Here's how the part is built. I have some questions about the finished solid (model axes, mm). A direction names the side the tool comes from. Coordinates: 2 decimals unless noted, no trailing zeros. Write each loop counter-clockwise with the first axis right and the second up, starting at its lowest first coordinate (ties: lowest second). Pieces come first, ordered by that corner, then holes. Notation, with made-up numbers: M -17.75,16 L 21.25,16 A33 cw 21.25,48 Z; hole C -17,42 d9. An arc over 180 degrees is marked long. Write each question's results on one line, items separated by ' | '. Start each with the question number.
from build123d import *

# Parameters (mm, degrees)
SKETCH_1_W          = 56.4
SKETCH_1_H          = 56.4
SKETCH_1_R          = 2.5
EXTRUDE_1_DEPTH     = 54.5
SKETCH_2_R          = 4
EXTRUDE_2_DEPTH     = 22
CUT_EXTRUDE_START   = -18
CUT_EXTRUDE_1_DEPTH = 18
SKETCH_4_R          = 19.05
EXTRUDE_3_DEPTH     = 2
CUT_EXTRUDE_2_DEPTH = 49.5


with BuildPart() as part:
    # 草图1 → 凸台-拉伸1 (new body)
    with BuildSketch(Plane.XY):
        Rectangle(SKETCH_1_W, SKETCH_1_H)
        with Locations((23.55, -23.55)):
            Circle(SKETCH_1_R, mode=Mode.SUBTRACT)
        with Locations((-23.55, -23.55)):
            Circle(SKETCH_1_R, mode=Mode.SUBTRACT)
        with Locations((23.55, 23.55)):
            Circle(SKETCH_1_R, mode=Mode.SUBTRACT)
        with Locations((-23.55, 23.55)):
            Circle(SKETCH_1_R, mode=Mode.SUBTRACT)
    extrude(amount=EXTRUDE_1_DEPTH)

    # 草图2 → 凸台-拉伸2 (add)
    with BuildSketch(Plane(origin=(0, 0, 0), x_dir=(-1, 0, 0), z_dir=(0, 0, -1))):
        Circle(SKETCH_2_R)
    extrude(amount=EXTRUDE_2_DEPTH)

    # 草图3 → 切除-拉伸1 (cut)
    with BuildSketch(Plane(origin=(0, 0, -22), x_dir=(-1, 0, 0), z_dir=(0, 0, -1)).offset(CUT_EXTRUDE_START)):
        with BuildLine():
            Line((1.936491673, -3.5), (-1.936491673, -3.5))
            ThreePointArc((-1.936491673, -3.5), (0, -4), (1.936491673, -3.5))
        make_face()
    extrude(amount=CUT_EXTRUDE_1_DEPTH, mode=Mode.SUBTRACT)

    # 草图4 → 凸台-拉伸3 (add)
    with BuildSketch(Plane(origin=(0, 0, 0), x_dir=(-1, 0, 0), z_dir=(0, 0, -1))):
        Circle(SKETCH_4_R)
    extrude(amount=EXTRUDE_3_DEPTH)

    # 草图5 → 切除-拉伸2 (cut)
    with BuildSketch(Plane.XY.offset(54.5)):
        with BuildLine():
            Line((23.57, 18.94), (28.2, 18.94))
            Line((28.2, 18.94), (28.2, 28.2))
            Line((28.2, 28.2), (18.94, 28.2))
            Line((18.94, 28.2), (18.94, 23.57))
            ThreePointArc((18.94, 23.57), (20.296095603, 20.296095603), (23.57, 18.94))
        make_face()
        with BuildLine():
            Line((18.94, -23.57), (18.94, -28.2))
            Line((18.94, -28.2), (28.2, -28.2))
            Line((28.2, -28.2), (28.2, -18.94))
            Line((28.2, -18.94), (23.57, -18.94))
            ThreePointArc((23.57, -18.94), (20.296095603, -20.296095603), (18.94, -23.57))
        make_face()
        with BuildLine():
            Line((-23.57, -18.94), (-28.2, -18.94))
            Line((-28.2, -18.94), (-28.2, -28.2))
            Line((-28.2, -28.2), (-18.94, -28.2))
            Line((-18.94, -28.2), (-18.94, -23.57))
            ThreePointArc((-18.94, -23.57), (-20.296095603, -20.296095603), (-23.57, -18.94))
        make_face()
        with BuildLine():
            Line((-18.94, 23.57), (-18.94, 28.2))
            Line((-18.94, 28.2), (-28.2, 28.2))
            Line((-28.2, 28.2), (-28.2, 18.94))
            Line((-28.2, 18.94), (-23.57, 18.94))
            ThreePointArc((-23.57, 18.94), (-20.296095603, 20.296095603), (-18.94, 23.57))
        make_face()
    extrude(amount=-CUT_EXTRUDE_2_DEPTH, mode=Mode.SUBTRACT)


solid = part.part
1) For pin 1 Ø3 at (x, y) = (-23.55, -23.55) entering from -Z; pin 2 Ø3 at (x, y) = (22, -22.5) entering from +Z; pin 3 Ø5 at (x, z) = (26, 27.5) entering from -Y; pin 4 Ø2.5 at (y, z) = (-26.5, 27.5) entering from -X, each with a flat end and sliding along its axis, tell me the tip position at first contact or that it passes through.
2) We'd pull the mould along Y, two halves only. Please class faces 5 (the flat face through (0, 0, 54.5)), 6 (the cylindrical face through (23.01, -25.99, 2.46)), 7 (the flat face through (0, 28.2, 27)), 8 (the flat face through (-26, -18.94, 30)): pulls with the +Y half, pulls with the -Y half, needs draft (parallel to the pull), parting line crosses it, or undercut.
3) I want a section at D-D, the plane z = 45. Write out the boundary of the cut face in (x, y), then the cut area to 3 significant figures.
4) I want a section at B-B, the plane y = 0. Write out the boundary of the cut face in (x, z), then the cut area to 3 significant figures.
5) For faces 1 (the flat face through (-0.4, 19.2, 0)), 2 (the flat face through (-26, -26, 5)), 3 (the flat face through (-18.94, 26, 30)), 4 (the flat face through (26, -26, 5)), which set-ups out of +Z, -Z, +X, -X, +Y, -Y let a thin tool reach every point of the face, with its end or its side?
6) I want a section at A-A, the plane z = 4. Write out the boundary of the cut face in (x, y).
7) Please list where these lines run through material, in increasing order: line 1 (X direction, y = 23.55, z = 1.95); line 2 (Z direction, x = -9.5, y = -9.5). Write a range as [from, to].
8) I want a section at C-C, the plane x = 0. Write out the boundary of the cut face in (y, z), then the cut area to 3 significant figures.
Output:
1) pin 1: passes through | pin 2: stops at z = 5 | pin 3: stops at y = -18.94 | pin 4: stops at x = -18.94
2) face 5: needs draft | face 6: undercut | face 7: pulls with the +Y half | face 8: pulls with the -Y half
3) outline: M -28.2,-18.94 L -23.57,-18.94 A4.63 cw -18.94,-23.57 L -18.94,-28.2 L 18.94,-28.2 L 18.94,-23.57 A4.63 cw 23.57,-18.94 L 28.2,-18.94 L 28.2,18.94 L 23.57,18.94 A4.63 cw 18.94,23.57 L 18.94,28.2 L -18.94,28.2 L -18.94,23.57 A4.63 cw -23.57,18.94 L -28.2,18.94 Z | area: 2,860 mm2
4) outline: M -28.2,0 L -19.05,0 L -19.05,-2 L -4,-2 L -4,-22 L 4,-22 L 4,-2 L 19.05,-2 L 19.05,0 L 28.2,0 L 28.2,54.5 L -28.2,54.5 Z | area: 3,310 mm2
5) face 1: -Z | face 2: +Z, -X, -Y | face 3: +Z, -X, +Y | face 4: +Z, +X, -Y
6) outline: M -28.2,-28.2 L 28.2,-28.2 L 28.2,28.2 L -28.2,28.2 Z; hole C -23.55,-23.55 d5; hole C -23.55,23.55 d5; hole C 23.55,-23.55 d5; hole C 23.55,23.55 d5
7) line 1: x = [-28.2, -26.05], [-21.05, 21.05], [26.05, 28.2] | line 2: z = [-2, 54.5]
8) outline: M -28.2,0 L -19.05,0 L -19.05,-2 L -4,-2 L -4,-4 L -3.5,-4 L -3.5,-22 L 4,-22 L 4,-2 L 19.05,-2 L 19.05,0 L 28.2,0 L 28.2,54.5 L -28.2,54.5 Z | area: 3,300 mm2
